Part model, mm, in its own coordinate system. Face numbers are marked on the shaded views. A direction names the side the tool comes from. Round coordinates to 2 decimals unless told otherwise and drop trailing zeros. Write each loop counter-clockwise with the first axis right and the second up, starting at its lowest first coordinate (ties: lowest second). Pieces come first, ordered by that corner, then holes. Notation, with made-up numbers: M 40.5,-26.75 L 61.5,-26.75 A17 cw 61.5,3.25 Z; hole C -32,83.5 d4. An arc over 180 degrees is marked long. One line per question, with ' | ' between items. Start each with the question number.
1) Drop flat-ended pins along their axis: pin 1 Ø5 at (x, z) = (23, 28) entering from -Y; pin 2 Ø3 at (y, z) = (5, 15) entering from -X; pin 3 Ø1 at (x, y) = (-18.5, 34.5) entering from +Z; pin 4 Ø10 at (x, z) = (-35, 24.5) entering from +Y. Give the stop position or say it passes through.
2) Tool access for the marked faces 1 and 2: list every direction of +Z, -Z, +X, -X, +Y, -Y with a clear straight run to the whole face (end or side of a thin tool).
3) Wall check: probe 1 along Z at (x, y) = (-19, -35); probe 2 along Z at (x, y) = (-25, 13); probe 3 along Y at (x, z) = (-9, 35). Give the ranges that are in metal, low to high. Write a range as [from, to].
4) Saw through at C-C (y = -39). List the corners of the cut face in (x, z), plus the area to 3 significant figures.
5) Saw through at D-D (x = -28). List the corners of the cut face in (y, z).
6) Saw through at A-A (x = 0). List the corners of the cut face in (y, z), plus the area to 3 significant figures.
7) Saw through at B-B (z = 46). List the corners of the cut face in (x, y), plus the area to 3 significant figures.
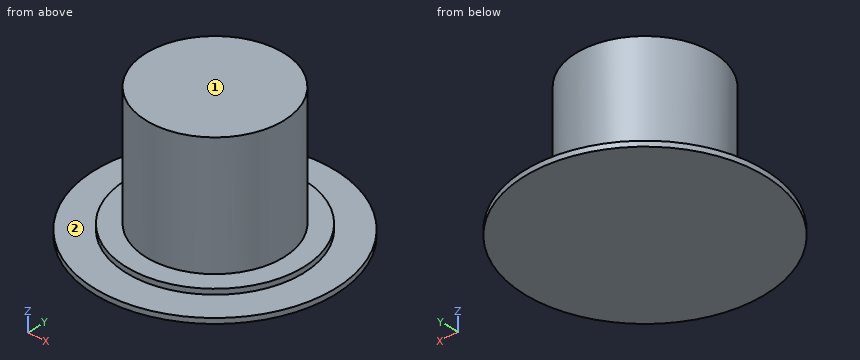
```python
from build123d import *

# Parameters (mm, degrees)
F0_R     = 45.491537
F3_DEPTH = 2
F1_R     = 33.53132
F4_DEPTH = 4
F2_R     = 26.021397
F5_DEPTH = 50


with BuildPart() as f3:
    # F0 (on Top) → F3 (new body)
    with BuildSketch(Plane.XY):
        Circle(F0_R)
    extrude(amount=F3_DEPTH)

    # F1 (on Top) → F4 (join)
    with BuildSketch(Plane.XY):
        Circle(F1_R)
    extrude(amount=F4_DEPTH)

    # F2 (on Top) → F5 (join)
    with BuildSketch(Plane.XY):
        Circle(F2_R)
    extrude(amount=F5_DEPTH)


solid = f3.part
```
Answer key:
1) pin 1: stops at y = -16.03 | pin 2: stops at x = -25.78 | pin 3: stops at z = 2 | pin 4: passes through
2) face 1: +Z, +X, -X, +Y, -Y | face 2: +Z
3) probe 1: z = [0, 2] | probe 2: z = [0, 4] | probe 3: y = [-24.42, 24.42]
4) outline: M -23.42,0 L 23.42,0 L 23.42,2 L -23.42,2 Z | area: 93.7 mm2
5) outline: M -35.85,0 L 35.85,0 L 35.85,2 L 18.45,2 L 18.45,4 L -18.45,4 L -18.45,2 L -35.85,2 Z
6) outline: M -45.49,0 L 45.49,0 L 45.49,2 L 33.53,2 L 33.53,4 L 26.02,4 L 26.02,50 L -26.02,50 L -26.02,4 L -33.53,4 L -33.53,2 L -45.49,2 Z | area: 2,710 mm2
7) outline: C 0,0 d52.04 | area: 2,130 mm2
